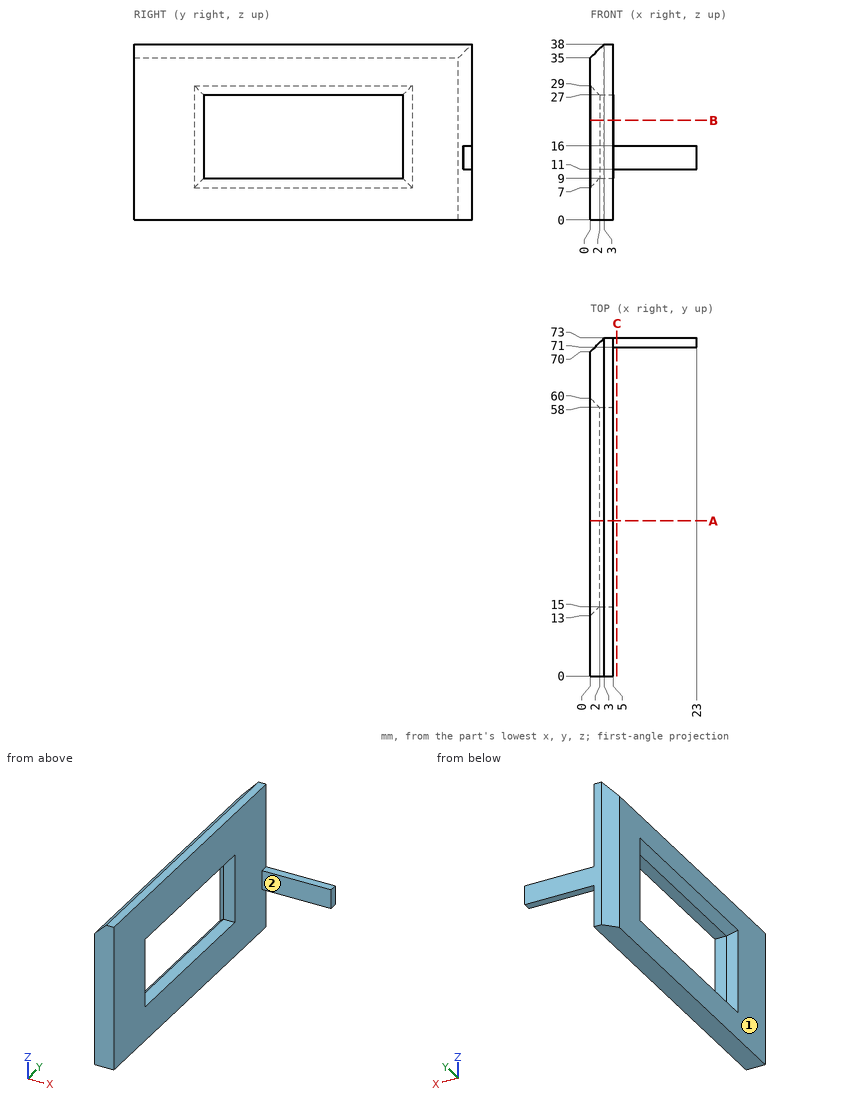
Design review of the part shown in the three views and the two pictorial views. Dimensions are in mm from the part's minimum x, y and z. A direction names the side the tool comes from. Give positions to 0.01 mm unless a question says otherwise; leave off trailing zeros. Write each loop counter-clockwise with the first axis right and the second up, starting at its lowest first coordinate (ties: lowest second). Pieces come first, ordered by that corner, then holes. Notation, with made-up numbers: M -24.75,36 L 9.25,36 A21 ccw 9.25,46 Z; hole C -22.75,-34.5 d3. An arc over 180 degrees is marked long. One line per item, written item: value.
1) For the marked faces 1 and 2, list the 3-axis set-ups (+Z, -Z, +X, -X, +Y, -Y) from which the entire face can be reached by the end or side of a thin tool; tool diameter is ignored.
Results are:
face 1: +Z, -Z, -X, +Y, -Y
face 2: +Z, -Z, +X, -Y
2) Take a section at B-B, the plane z = 21.5. Write out the cut boundary in (x, y).
Results are:
outline: M 0,0 L 5,0 L 5,15 L 2,15 L 0,13 Z; M 0,60 L 2,58 L 5,58 L 5,73 L 3,73 L 0,70 Z
3) Take a section at A-A, the plane y = 33.5. Write out the cut boundary in (x, z).
Results are:
outline: M 0,0 L 5,0 L 5,9 L 2,9 L 0,7 Z; M 0,29 L 2,27 L 5,27 L 5,38 L 3,38 L 0,35 Z
4) For line 1 (Z direction, x = 4.25, y = 39); line 2 (X direction, y = 49.5, z = 32); line 3 (Y direction, x = 8, z = 11.5), list the stretches that pass through material, from the lowest coordinate up. Write a range as from..to.
Results are:
line 1: z = 0..9, 27..38
line 2: x = 0..5
line 3: y = 71..73
5) Take a section at C-C, the plane x = 5.75. Write out the cut boundary in (y, z).
Results are:
outline: M 71,11 L 73,11 L 73,16 L 71,16 Z
6) For P1, Ø2, axis at x = 11, y = 72.5, coming from the -Z side; P2, Ø6, axis at y = 34, z = 13.5, coming from the -X side; P3, Ø2.5, axis at x = 14, z = 13.5, coming from the -Y side; P4, Ø1.6, axis at x = 13, y = 72.5, coming from the +Z side, all flat-tipped, find the tip position at first contact; note any pin that passes through.
Results are:
P1: stops at z = 11
P2: passes through
P3: stops at y = 71
P4: stops at z = 16
